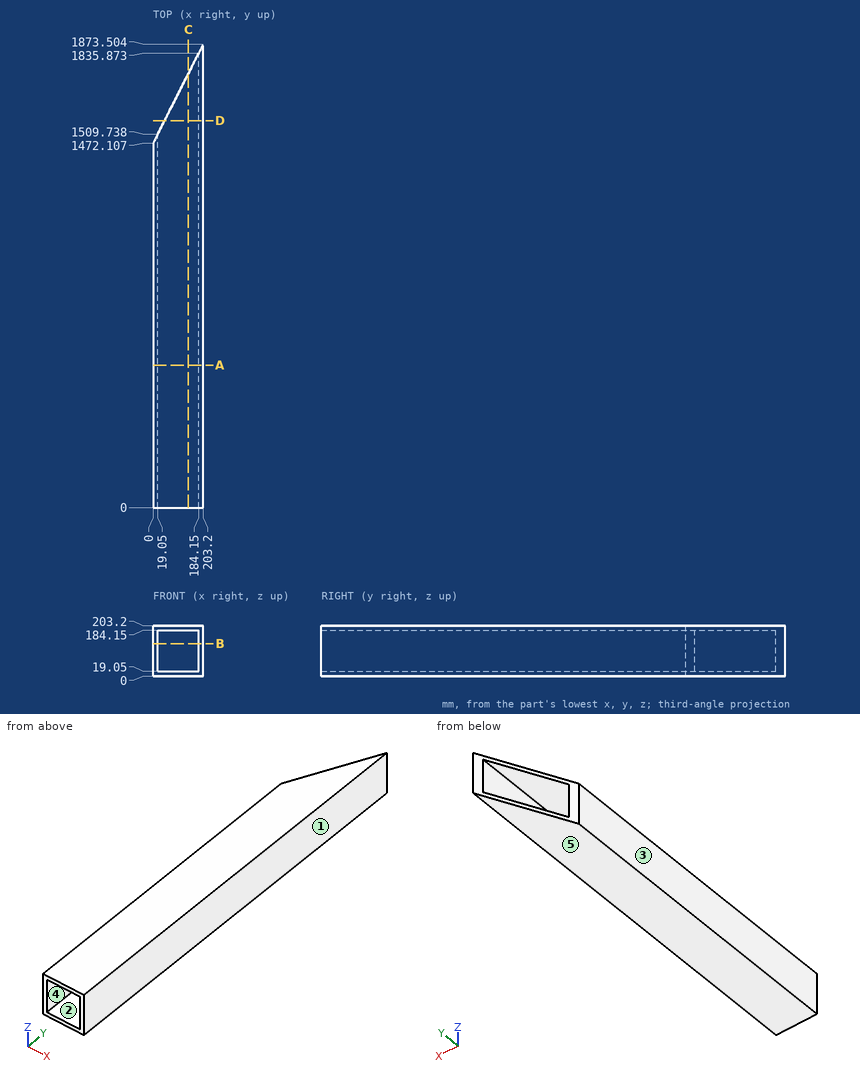
Study the drawing (mm; zero at the part's minimum x, y, z) and answer. A direction names the side the tool comes from. Give positions to 0.01 mm unless a question says otherwise; leave off trailing zeros. Order: outer loops, then holes, each group sorted by start corner. A loop starts at its lowest first (then second) coordinate and runs counter-clockwise, first axis right, second up.
1. Section B-B, the plane z = 130.5 is taken. Determine the outline of the cut face in (x, y).
Result sheet:
outline: (0, 0) - (19.05, 0) - (19.05, 1509.74) - (0, 1472.11) - close; (184.15, 0) - (203.2, 0) - (203.2, 1873.5) - (184.15, 1835.87) - close
2. The mould has two halves that part along Z. Classify the marked faces 3, 4 and 5: released by +Z, released by -Z, zero draft, split by the parting line, or undercut.
Result sheet:
face 3: zero draft
face 4: undercut
face 5: released by -Z
3. Section A-A, the plane y = 576.5 is taken. Determine the outline of the cut face in (x, z), and give its area (3 significant figures).
Result sheet:
outline: (0, 0) - (203.2, 0) - (203.2, 203.2) - (0, 203.2) - close; hole (19.05, 19.05) - (184.15, 19.05) - (184.15, 184.15) - (19.05, 184.15) - close
area: 14,000 mm2
4. Section C-C, the plane x = 143 is taken. Determine the outline of the cut face in (y, z), and give its area (4 significant figures).
Result sheet:
outline: (0, 0) - (1754.59, 0) - (1754.59, 19.05) - (0, 19.05) - close; (0, 184.15) - (1754.59, 184.15) - (1754.59, 203.2) - (0, 203.2) - close
area: 66,850 mm2
5. For the marked faces 1 and 2, determine the directions among +Z, -Z, +X, -X, +Y, -Y from which every point of the face is accessible in a straight line to the end or side of a thin tool.
Result sheet:
face 1: +Z, -Z, +X, +Y, -Y
face 2: +Y, -Y
6. Section D-D, the plane y = 1563.5 is taken. Determine the outline of the cut face in (x, z), and give its area (3 significant figures).
Result sheet:
outline: (46.27, 0) - (203.2, 0) - (203.2, 203.2) - (46.27, 203.2) - (46.27, 184.15) - (184.15, 184.15) - (184.15, 19.05) - (46.27, 19.05) - close
area: 9,120 mm2
7. Straight lines are drawn through the part: L1, parallel to Z at x = 82.5, y = 1431; L2, parallel to Y at x = 187.5, z = 108. For each, find the intervals that lie inside material, in ascending order.
Result sheet:
L1: z = 0 to 19.05, 184.15 to 203.2
L2: y = 0 to 1842.49
